Build history of the part. All positions in model axes, mm. Face numbers are marked on the shaded views. A direction names the side the tool comes from. Give positions to 0.01 mm unless a question says otherwise; leave off trailing zeros. Order: outer loops, then holes, each group sorted by start corner. A loop starts at its lowest first (then second) coordinate and runs counter-clockwise, first axis right, second up. Notation, with made-up numbers: M 36,48 L 90,48 A15 cw 90,54 Z; hole C 71,73.25 d4. An arc over 180 degrees is marked long. Use CSV: the item, a comma, the result in double quotes. Start each with the question number.
Item 1: Wall check: line 1 along X through (y, z) = (-10, -10.5); line 2 along Z through (x, y) = (0, 21); line 3 along Z through (x, y) = (19, 0). Give the ranges that are in metal, low to high.
Item 2: Band-saw the part on B-B on y = 0. Write the cut outline in (x, z), plus the area to 3 significant figures.
Item 3: Band-saw the part on D-D on y = 19. Write the cut outline in (x, z).
Item 4: Pin check, flat tips, straight feed: P1, Ø1.5, axis at y = 23, z = -2, coming from the +X side; P2, Ø12, axis at x = 31, y = -17, coming from the +Z side; P3, Ø6, axis at y = -17, z = 13, coming from the -X side. Stop position of each tip, or through.
Item 5: Band-saw the part on A-A on x = 0. Write the cut outline in (y, z), plus the area to 3 significant figures.
Item 6: Two-plate mould, pull along X, no slides. Class the marked faces 1, 2, 3 and 4: pulls with the +X half, pulls with the -X half, needs draft (parallel to the pull), parting line crosses it, or undercut.
Item 7: Which spindle directions (+Z, -Z, +X, -X, +Y, -Y) get a long thin tool onto all of the face, cutting with end or side? Do the marked faces 5, 6, 7 and 8. Say none if no direction does.
Item 8: Band-saw the part on C-C on x = 13. Write the cut outline in (y, z).
Autodesk Inventor part; units mm, degrees
ref_plane "YZ Plane" through (0, 0, 0) normal (1, 0, 0) x (0, 1, 0)
ref_plane "XZ Plane" through (0, 0, 0) normal (0, 1, 0) x (-1, 0, 0)
ref_plane "XY Plane" through (0, 0, 0) normal (0, 0, 1) x (1, 0, 0)
sketch "Sketch1" plane through (0, 0, 0) normal (0, 0, 1) x (1, 0, 0)
  line L0 (-20, 23.5) -> (20, 23.5)
  line L1 (20, 23.5) -> (20, -23.5)
  line L2 (20, -23.5) -> (-20, -23.5)
  line L3 (-20, -23.5) -> (-20, 23.5)
  line L4 (-12, 15) -> (12, 15)
  line L5 (12, 15) -> (12, -15)
  line L6 (12, -15) -> (-12, -15)
  line L7 (-12, -15) -> (-12, 15)
  point P0 (0, 0)
  point P1 (20, 0)
  point P2 (0, 23.5)
  point P3 (12, 0)
  point P4 (0, 15)
  dimension "d0" = 40
  dimension "d1" = 47
  dimension "d2" = 24
  dimension "d12" = 30
extrude "Extrusion1" add sketch "Sketch1" along normal mid plane 46
sketch "Sketch2" plane through (0, 0, 0) normal (1, 0, 0) x (0, 1, 0)
  circle A0 centre (0, 0) radius 9
  circle A1 centre (0, 0) radius 18
  dimension "d5" = 18
  dimension "d6" = 36
extrude "Extrusion2" cut sketch "Sketch2" along normal through all both and the other way through all contours A0
extrude "Extrusion3" add sketch "Sketch2" along normal blind 22 from surface at 20
mirror "Mirror1" about plane through (0, 0, 0) normal (1, 0, 0) of "Extrusion3"
sketch "Sketch3" plane through (-20, 23.5, 23) normal (0, 1, 0) x (1, 0, 0)
  circle A0 centre (20, 23) radius 7.5
  circle A1 centre (20, 23) radius 15
  dimension "d13" = 15
  dimension "d14" = 30
extrude "Extrusion4" cut sketch "Sketch3" against normal through all contours A0
extrude "Extrusion5" add sketch "Sketch3" along normal blind 10
mirror "Mirror2" about plane through (0, 0, 0) normal (0, 1, 0) of "Extrusion5"
ref_plane "Work Plane1" through (0, 0, 0) normal (0, 1, 0) x (-1, 0, 0)
properties part number "DP816"
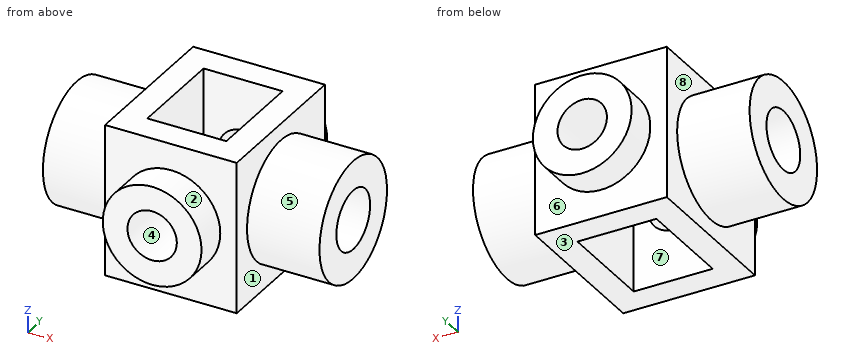
Model answer:
1,line 1,"x = -42 to -12, 12 to 42"
1,line 2,"z = -23 to -7.5, 7.5 to 23"
1,line 3,"z = -23 to -9, 9 to 23"
2,outline,"M -42,-18 L -20,-18 L -20,-23 L -12,-23 L -12,-9 L -42,-9 Z; M -42,9 L -12,9 L -12,23 L -20,23 L -20,18 L -42,18 Z; M 12,-23 L 20,-23 L 20,-18 L 42,-18 L 42,-9 L 12,-9 Z; M 12,9 L 42,9 L 42,18 L 20,18 L 20,23 L 12,23 Z"
2,area,"1,240 mm^2"
3,outline,"M -20,-23 L 20,-23 L 20,23 L -20,23 Z; hole C 0,0 d15"
4,P1,"stops at x = 20"
4,P2,"stops at z = 14.25"
4,P3,"stops at x = -20"
5,outline,"M -33.5,-15 L -23.5,-15 L -23.5,-23 L -15,-23 L -15,-7.5 L -33.5,-7.5 Z; M -33.5,7.5 L -15,7.5 L -15,23 L -23.5,23 L -23.5,15 L -33.5,15 Z; M 15,-23 L 23.5,-23 L 23.5,-15 L 33.5,-15 L 33.5,-7.5 L 15,-7.5 Z; M 15,7.5 L 33.5,7.5 L 33.5,15 L 23.5,15 L 23.5,23 L 15,23 Z"
5,area,"827 mm^2"
6,face 1,"pulls with the +X half"
6,face 2,"parting line crosses it"
6,face 3,"needs draft"
6,face 4,"undercut"
7,face 5,"+X"
7,face 6,"+Y"
7,face 7,"+Z, -Z"
7,face 8,"-X"
8,outline,"M -33.5,-7.48 L -23.5,-7.48 L -23.5,-23 L 23.5,-23 L 23.5,-7.48 L 33.5,-7.48 L 33.5,7.48 L 23.5,7.48 L 23.5,23 L -23.5,23 L -23.5,7.48 L -33.5,7.48 Z; hole C 0,0 d18"
